Check sheet for the drawn part. Datum: minimum x, y, z corner. Units: mm. A direction names the side the tool comes from. Give positions to 0.01 mm unless a question says otherwise; leave off trailing zeros. Write each loop counter-clockwise with the first axis right and the second up, starting at its lowest first coordinate (ties: lowest second). Pieces come first, ordered by that corner, then holes.
(1) Cross-section at C-C (z = 76.2). Record the boundary of the cut face in (x, y).
(2) Mould release check, pull along X, two halves, no side actions. Record for the marked faces 3, 4, 5 and 6: +X half, -X half, draft (parallel to the pull), parting line (faces both ways), or undercut.
(3) Cross-section at D-D (y = 60). Record the boundary of the cut face in (x, z).
(4) Depth check by flat-ended pin: P1, Ø5, axis at x = 23.5, z = 92.5, coming from the +Y side; P2, Ø1, axis at y = 74.5, z = 28, coming from the +X side; P3, Ø5, axis at y = 29.5, z = 43.5, coming from the +X side. Enter the tip coordinate at first touch or a pass-through.
(5) Cross-section at B-B (y = 38.1). Record the boundary of the cut face in (x, z), and give its area (3 significant figures).
(6) Tool access check on the marked faces 1 and 2. Record the directions out of +Z, -Z, +X, -X, +Y, -Y that give a thin tool (end or side, any length) a straight path to the whole face; none if there is none.
(7) Cross-section at A-A (x = 152.4). Record the boundary of the cut face in (y, z).
(8) Thickness scan on line 1 along Z through (x, y) = (93, 38); line 2 along Z through (x, y) = (37.5, 39); line 3 along Y through (x, z) = (35, 96.5). Record the ranges inside material, lowest first.
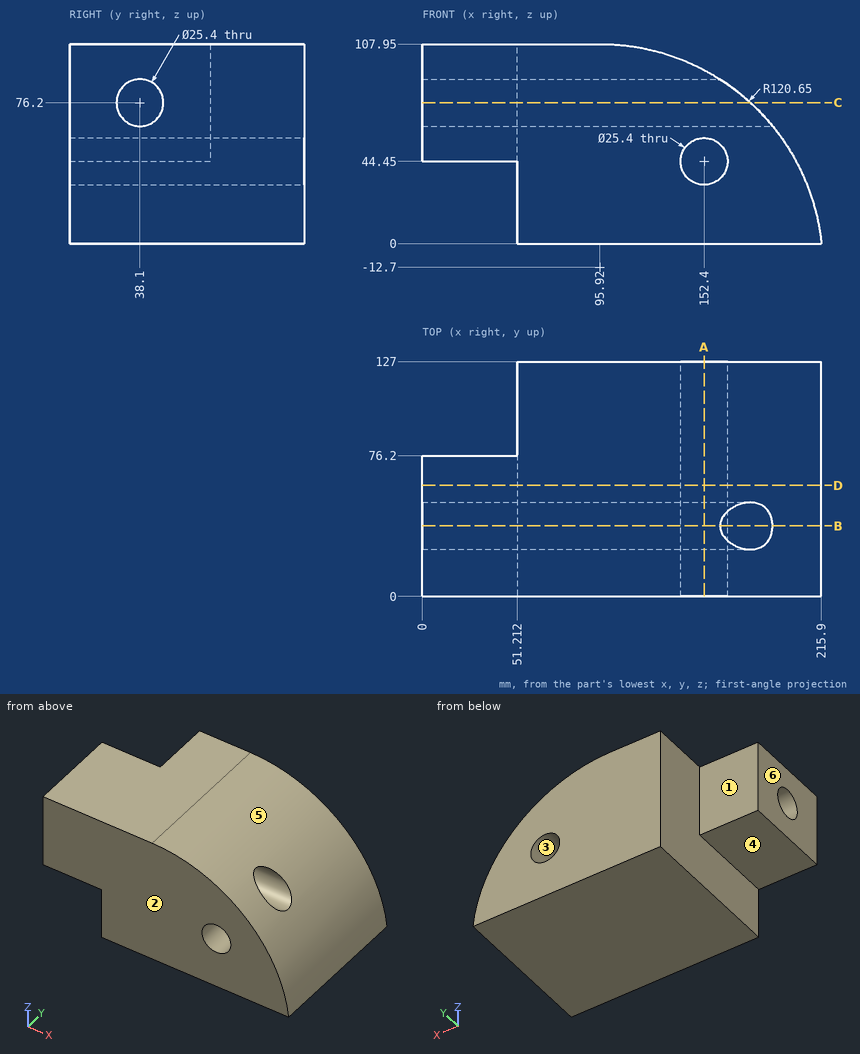
Reply:
1. outline: (0, 0) - (177.49, 0) - (177.49, 25.4) - (0, 25.4) - close; (0, 50.8) - (177.49, 50.8) - (177.49, 127) - (51.21, 127) - (51.21, 76.2) - (0, 76.2) - close
2. face 3: undercut
2. face 4: draft
2. face 5: +X half
2. face 6: -X half
3. outline: (0, 44.45) - (51.21, 44.45) - (51.21, 0) - (215.9, 0) arc R120.65 ccw to (95.92, 107.95) - (0, 107.95) - close; hole circle Ø25.4 at (152.4, 44.45)
4. P1: stops at y = 76.2
4. P2: stops at x = 209.68
4. P3: stops at x = 203.96
5. outline: (0, 44.45) - (51.21, 44.45) - (51.21, 0) - (215.9, 0) arc R120.65 ccw to (189.46, 63.5) - (0, 63.5) - close; (0, 88.9) - (160.99, 88.9) arc R120.65 ccw to (95.92, 107.95) - (0, 107.95) - close; hole circle Ø25.4 at (152.4, 44.45)
5. area: 13,000 mm2
6. face 1: +Z, -Z, -X, +Y
6. face 2: +Z, -Z, +X, -X, -Y
7. outline: (0, 0) - (127, 0) - (127, 31.75) - (0, 31.75) - close; (0, 57.15) - (127, 57.15) - (127, 93.91) - (0, 93.91) - close; hole circle Ø25.4 at (38.1, 76.2)
8. line 1: z = 0 to 63.5, 88.9 to 107.95
8. line 2: z = 44.45 to 63.53, 88.87 to 107.95
8. line 3: y = 0 to 76.2
